from build123d import *

# Parameters (mm, degrees)
BOSS_EXTRUDE1_DEPTH = 2.9
SKETCH2_R           = 3.5
BOSS_EXTRUDE2_DEPTH = 5
FILLET1_R           = 1
FILLET2_R           = 0.2
M4_TAPPED_HOLE1_D   = 3.3


with BuildPart() as part:
    # Sketch1 → Boss-Extrude1 (new body)
    with BuildSketch(Plane(origin=(0, 0, 0), x_dir=(1, 0, 0), z_dir=(0, 1, 0))):
        Polygon((4.041451884, 0), (2.020725942, 3.5), (-2.020725942, 3.5), (-4.041451884, 0), (-2.020725942, -3.5), (2.020725942, -3.5), align=None)
    extrude(amount=BOSS_EXTRUDE1_DEPTH)

    # Sketch2 → Boss-Extrude2 (add)
    with BuildSketch(Plane.XZ):
        Circle(SKETCH2_R)
    extrude(amount=-BOSS_EXTRUDE2_DEPTH)

    # Fillet1
    fillet1_edges = [part.edges().sort_by_distance(p)[0] for p in [
        (-3.5, 5, 0),
    ]]
    fillet(fillet1_edges, radius=FILLET1_R)

    # Fillet2
    fillet2_edges = [part.edges().sort_by_distance(p)[0] for p in [
        (2.020725942, 1.45, 3.5),
        (-2.020725942, 1.45, 3.5),
        (-4.041451884, 1.45, 0),
        (-2.020725942, 1.45, -3.5),
        (2.020725942, 1.45, -3.5),
        (4.041451884, 1.45, 0),
    ]]
    fillet(fillet2_edges, radius=FILLET2_R)

    # M4 Tapped Hole1 (through all)
    with Locations(Plane(origin=(0, 0, 0), x_dir=(-1, 0, 0), z_dir=(0, -1, 0))):
        with Locations((0, 0)):
            Hole(M4_TAPPED_HOLE1_D / 2)


solid = part.part
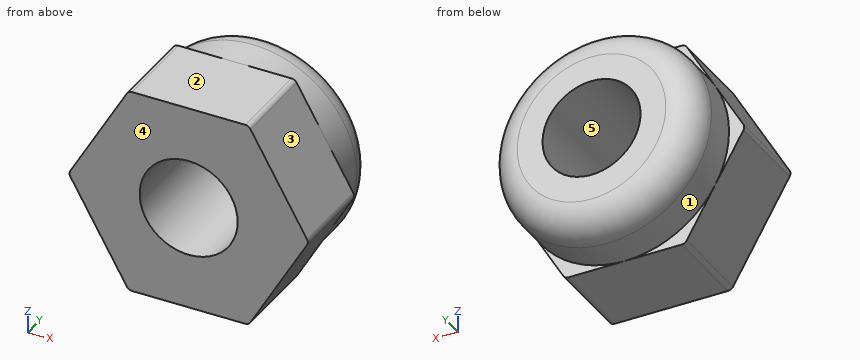
Could you check a few things on this model? Use its own coordinates, in mm. Face numbers are marked on the shaded views. A direction names the side the tool comes from. Give positions to 0.01 mm unless a question says otherwise; leave off trailing zeros. Order: outer loops, then holes, each group sorted by start corner. A loop starts at its lowest first (then second) coordinate and runs counter-clockwise, first axis right, second up. Notation, with made-up numbers: (-34, 86) -> (-16, 86) arc R33 cw to (-16, 115) -> close; hole circle Ø1 at (-7.75, 67). An arc over 180 degrees is marked (long way). Answer in a Markdown table with one row per item. Add a question column.
Item 1: Imagine slicing it at D-D (y = 4.45). List the corners of the cut face in (x, z) for me, and give its area (3 significant figures).
Item 2: Imagine slicing it at C-C (y = 3.65). List the corners of the cut face in (x, z) for me, and give its area (3 significant figures).
Item 3: Imagine slicing it at B-B (y = 1.5). List the corners of the cut face in (x, z) for me.
Item 4: I'm going to push flat-ended pins straight in: P1, Ø1, axis at y = 1, z = 1.5, coming from the -X side; P2, Ø0.5, axis at x = -3.5, z = 0, coming from the +Y side; P3, Ø0.8, axis at x = 3.5, z = -0.5, coming from the +Y side. Where does each tip first touch, or does it pass through?
Item 5: For the marked faces 1 and 2, which set-ups out of +Z, -Z, +X, -X, +Y, -Y let a thin tool reach every point of the face, with its end or its side?
Item 6: We'd pull the mould along X, two halves only. Please class the marked faces 3, 4 and 5: pulls with the +X half, pulls with the -X half, needs draft (parallel to the pull), parting line crosses it, or undercut.
Item 7: Imagine slicing it at A-A (z = 0). List the corners of the cut face in (x, y) for me, and give its area (3 significant figures).
Item 8: Please list where these lines run through material, in increasing order: probe 1 along Z at (x, y) = (0, 2); probe 2 along X at (y, z) = (1.9, -0.75); probe 3 along X at (y, z) = (4.1, -1.5).
Result:
| question | item | result |
|---|---|---|
| 1 | outline | circle Ø6.79 at (0, 0); hole circle Ø3.3 at (0, 0) |
| 1 | area | 27.6 mm2 |
| 2 | outline | circle Ø7 at (0, 0); hole circle Ø3.3 at (0, 0) |
| 2 | area | 29.9 mm2 |
| 3 | outline | (-3.98, -0.1) -> (-2.08, -3.4) arc R0.2 ccw to (-1.91, -3.5) -> (1.91, -3.5) arc R0.2 ccw to (2.08, -3.4) -> (3.98, -0.1) arc R0.2 ccw to (3.98, 0.1) -> (2.08, 3.4) arc R0.2 ccw to (1.91, 3.5) -> (-1.91, 3.5) arc R0.2 ccw to (-2.08, 3.4) -> (-3.98, 0.1) arc R0.2 ccw to start; hole circle Ø3.3 at (0, 0) |
| 4 | P1 | x = -3.46 |
| 4 | P2 | y = 4.66 |
| 4 | P3 | y = 4.77 |
| 5 | face 1 | +Y |
| 5 | face 2 | +Z, +X, -X, +Y, -Y |
| 6 | face 3 | pulls with the +X half |
| 6 | face 4 | needs draft |
| 6 | face 5 | undercut |
| 7 | outline | (-4.01, 0) -> (-1.65, 0) -> (-1.65, 5) -> (-2.5, 5) arc R1 ccw to (-3.5, 4) -> (-3.5, 2.9) -> (-4.01, 2.9) -> close; (1.65, 0) -> (4.01, 0) -> (4.01, 2.9) -> (3.5, 2.9) -> (3.5, 4) arc R1 ccw to (2.5, 5) -> (1.65, 5) -> close |
| 7 | area | 21.0 mm2 |
| 8 | probe 1 | -3.5 to -1.65, 1.65 to 3.5 |
| 8 | probe 2 | -3.61 to -1.47, 1.47 to 3.61 |
| 8 | probe 3 | -3.16 to -0.69, 0.69 to 3.16 |
